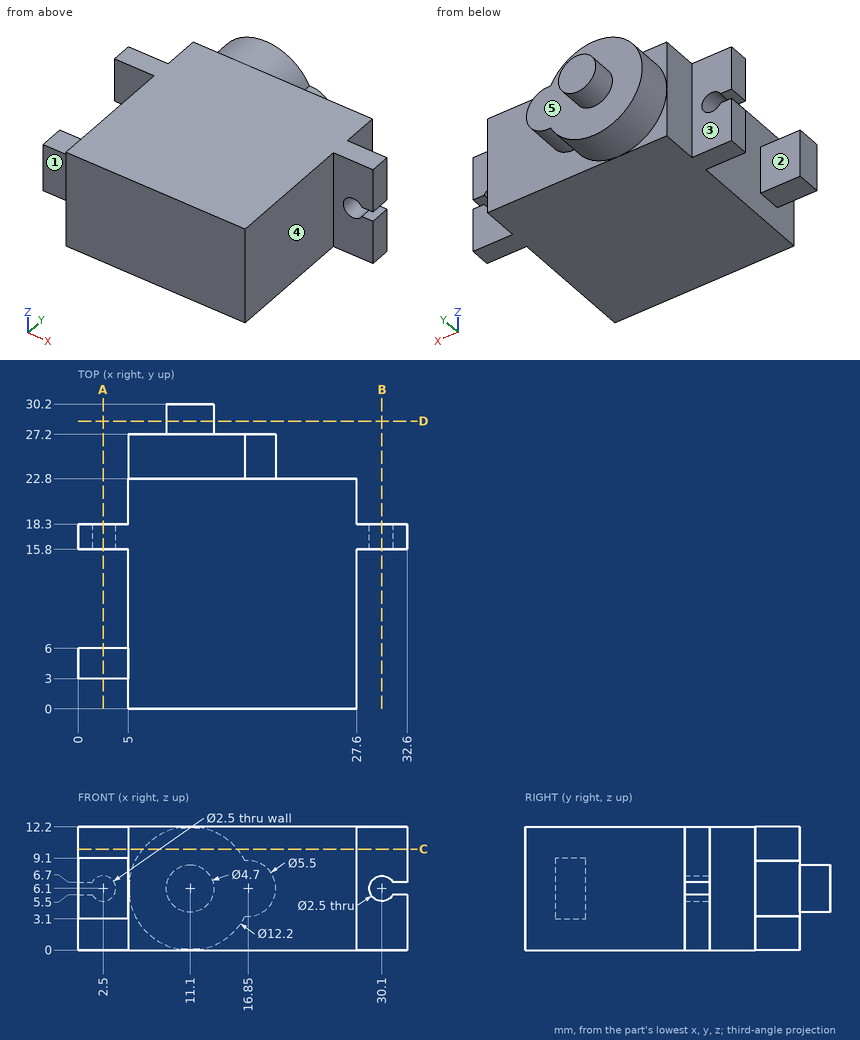
For this review, use the dimensioned drawing (mm, ordinates from the lowest corner) and the shaded views. A direction names the side the tool comes from. Give positions to 0.01 mm unless a question says otherwise; leave off trailing zeros. Write each loop counter-clockwise with the first axis right and the second up, starting at its lowest first coordinate (ties: lowest second). Pieces come first, ordered by that corner, then holes. Notation, with made-up numbers: M 59,3 L 66,3 A23 cw 66,18 Z; hole C 64.25,23 d1. An arc over 180 degrees is marked long. Answer as a JSON object with one key per item and string values. Group by question number.
1) We need section D-D (y = 28.5). Give the boundary of the cut face in (x, z), and give its area (3 significant figures).
2) We need section B-B (x = 30.1). Give the boundary of the cut face in (y, z), and give its area (4 significant figures).
3) Mouldability with a two-part tool opening along X and no side actions: class the marked faces 4 and 5 as released by +X, released by -X, zero draft, split by the parting line, or undercut.
4) For line 1 along X through (y, z) = (17.4, 6.1); line 2 along X through (y, z) = (9.5, 9.5); line 3 along Y through (x, z) = (23, 8.5), list the stretches that pass through material, from the lowest coordinate up.
5) Tool access review of the marked faces 1, 2 and 3: name each direction out of +Z, -Z, +X, -X, +Y, -Y from which nothing blocks a thin tool from reaching the whole face with its end or side.
6) We need section C-C (z = 10). Give the boundary of the cut face in (x, y).
7) Clearance check with flat-ended pins moving along their axes: pin 1 Ø3 at (x, y) = (7, 26.5) entering from +Z; pin 2 Ø5.5 at (x, z) = (1.5, 6.5) entering from -Y; pin 3 Ø1.5 at (x, z) = (30, 8) entering from -Y; pin 4 Ø2 at (x, z) = (30.1, 6.1) entering from -Y. State where each tip first meets the part, or that it passes through.
8) We need section A-A (x = 2.5). Give the boundary of the cut face in (y, z).
Answer key:
{
 "1": {"outline": "C 11.1,6.1 d4.7", "area": "17.3 mm²"},
 "2": {"outline": "M 15.8,0 L 18.3,0 L 18.3,4.85 L 15.8,4.85 Z; M 15.8,7.35 L 18.3,7.35 L 18.3,12.2 L 15.8,12.2 Z", "area": "24.25 mm²"},
 "3": {"face 4": "released by +X", "face 5": "zero draft"},
 "4": {"line 1": "x = 3.75 to 28.85", "line 2": "x = 5 to 27.6", "line 3": "y = 0 to 22.8"},
 "5": {"face 1": "+Z, -Z, -X, -Y", "face 2": "+Z, -Z, -X", "face 3": "+Z, -Z, -X, +Y"},
 "6": {"outline": "M 0,15.8 L 5,15.8 L 5,0 L 27.6,0 L 27.6,15.8 L 32.6,15.8 L 32.6,18.3 L 27.6,18.3 L 27.6,22.8 L 15.79,22.8 L 15.79,27.2 L 6.41,27.2 L 6.41,22.8 L 5,22.8 L 5,18.3 L 0,18.3 Z"},
 "7": {"pin 1": "stops at z = 11.62", "pin 2": "stops at y = 3", "pin 3": "stops at y = 15.8", "pin 4": "passes through"},
 "8": {"outline": "M 3,3.1 L 6,3.1 L 6,9.1 L 3,9.1 Z; M 15.8,0 L 18.3,0 L 18.3,4.85 L 15.8,4.85 Z; M 15.8,7.35 L 18.3,7.35 L 18.3,12.2 L 15.8,12.2 Z"}
}
